Autodesk Inventor part; units mm, degrees
ref_plane "YZ Plane" through (0, 0, 0) normal (1, 0, 0) x (0, 1, 0)
ref_plane "XZ Plane" through (0, 0, 0) normal (0, 1, 0) x (-1, 0, 0)
ref_plane "XY Plane" through (0, 0, 0) normal (0, 0, 1) x (1, 0, 0)
sketch "Sketch1" plane through (0, 0, 0) normal (0, 1, 0) x (-1, 0, 0)
  line L0 (1.27, 1.27) -> (-1.27, 1.27)
  line L1 (-1.27, 1.27) -> (-1.27, -1.27)
  line L2 (-1.27, -1.27) -> (1.27, -1.27)
  line L3 (1.27, -1.27) -> (1.27, 1.27)
  line L4 (1.27, 1.27) -> (-1.27, -1.27) construction
  line L5 (-1.27, 1.27) -> (1.27, -1.27) construction
  point P0 (0, 0)
  dimension "d0" = 2.54
  dimension "d1" = 2.54
extrude "Extrusion1" add sketch "Sketch1" along normal blind 2.6
fillet "Fillet1" radius 0.5 4 edges at (1.27, 1.3, 1.27) (1.27, 1.3, -1.27) (-1.27, 1.3, 1.27) (-1.27, 1.3, -1.27)
sketch "Sketch2" plane through (0, 2.6, 0) normal (0, 1, 0) x (1, 0, 0)
  line L0 (-0.3, -0.3) -> (0.3, -0.3)
  line L1 (0.3, -0.3) -> (0.3, 0.3)
  line L2 (0.3, 0.3) -> (-0.3, 0.3)
  line L3 (-0.3, 0.3) -> (-0.3, -0.3)
  line L4 (-0.3, -0.3) -> (0.3, 0.3) construction
  line L5 (0.3, -0.3) -> (-0.3, 0.3) construction
  point P0 (0, 0)
  dimension "d5" = 0.6
  dimension "d6" = 0.6
extrude "Extrusion2" add sketch "Sketch2" along normal blind 5.8
chamfer "Chamfer1" distance 0.2 angle 45 4 edges at (0.3, 8.4, 0) (0, 8.4, 0.3) (-0.3, 8.4, 0) (0, 8.4, -0.3)
sketch "Sketch3" plane through (0, 0, 0) normal (0, -1, 0) x (1, 0, 0)
  line L0 (0.3, 0.3) -> (-0.3, 0.3)
  line L1 (-0.3, 0.3) -> (-0.3, -0.3)
  line L2 (-0.3, -0.3) -> (0.3, -0.3)
  line L3 (0.3, -0.3) -> (0.3, 0.3)
  point P0 (0, 0)
extrude "Extrusion3" add sketch "Sketch3" along normal blind 2
fillet "Fillet2" radius 0.28 4 edges at (0, -2, -0.3) (-0.3, -2, 0) (0, -2, 0.3) (0.3, -2, 0)
properties part number "PIR pins"
Build history of the part. All positions in model axes, mm. Coordinates: 2 decimals unless noted, no trailing zeros. Order: outer loops, then holes, each group sorted by start corner. A loop starts at its lowest first (then second) coordinate and runs counter-clockwise, first axis right, second up. Notation, with made-up numbers: M 65.25,80.25 L 78.25,80.25 A19 cw 78.25,89.25 Z; hole C 63,27 d5. An arc over 180 degrees is marked long. One line per question, with ' | ' between items. Start each with the question number.
Q1. Saw through at C-C (x = -0.65). List the corners of the cut face in (y, z), then the cut area to 3 significant figures.
Q2. Saw through at A-A (y = 2). List the corners of the cut face in (x, z).
Q3. Saw through at B-B (z = 0.5). List the corners of the cut face in (x, y), then the cut area to 3 significant figures.
Q4. Probe L1, parallel to Y at x = 0.55, z = 0.75; L2, parallel to Z at x = 0.1, y = 3.75. List the from-to ranges inside material, lowest first. Write a range as from..to.
Q5. Flat gauge pins, fed straight in: pin 1 Ø0.5 at (x, y) = (0, -0.5) entering from +Z; pin 2 Ø1 at (x, z) = (1, 0) entering from -Y; pin 3 Ø1.5 at (x, z) = (-1, 0) entering from +Y. Where does each tip first touch, or does it go through?
Check values:
1) outline: M 0,-1.27 L 2.6,-1.27 L 2.6,1.27 L 0,1.27 Z | area: 6.60 mm2
2) outline: M -1.27,-0.77 A0.5 ccw -0.77,-1.27 L 0.77,-1.27 A0.5 ccw 1.27,-0.77 L 1.27,0.77 A0.5 ccw 0.77,1.27 L -0.77,1.27 A0.5 ccw -1.27,0.77 Z
3) outline: M -1.27,0 L 1.27,0 L 1.27,2.6 L -1.27,2.6 Z | area: 6.60 mm2
4) L1: y = 0..2.6 | L2: z = -0.3..0.3
5) pin 1: stops at z = 0.3 | pin 2: stops at y = 0 | pin 3: stops at y = 8.25
